from build123d import *

# Parameters (mm, degrees)
F0_R     = 25
F1_DEPTH = 1.2


with BuildPart() as f1:
    # F0 (on Top) → F1 (new body)
    with BuildSketch(Plane.XY):
        Circle(F0_R)
        Polygon((5, 15), (5, 5), (15, 5), (15, -5), (5, -5), (5, -15), (-5, -15), (-5, -5), (-15, -5), (-15, 5), (-5, 5), (-5, 15), align=None, mode=Mode.SUBTRACT)
    extrude(amount=F1_DEPTH)


solid = f1.part
For this review, take the finished solid that the model builds, in its own axes (mm). A direction names the side the tool comes from. Give positions to 0.01 mm unless a question says otherwise; leave off trailing zeros. Order: outer loops, then holes, each group sorted by start corner. A loop starts at its lowest first (then second) coordinate and runs counter-clockwise, first axis right, second up. Notation, with made-up numbers: M 61,81 L 83,81 A17 ccw 83,100 Z; hole C 80,63.25 d1. An arc over 180 degrees is marked long. Answer in a Markdown table with one row per item. Add a question column.
(1) Consider section C-C on z = 0.8. State the section outline as (x, y) points, and give its area (3 significant figures).
(2) For faces 1 (the face through (0, -15, 1)), 2 (the face through (5.2, -5.2, 0)), list the 3-axis set-ups (+Z, -Z, +X, -X, +Y, -Y) from which the entire face can be reached by the end or side of a thin tool; tool diameter is ignored.
(3) Wall thickness on probe 1 along X at (y, z) = (0.5, 1.05) (3 decimals); probe 2 along X at (y, z) = (2, 1.15); probe 3 along Y at (x, z) = (-3, 1.1): over which ranges is each line inside the solid? List them lowest first. Write a range as [from, to].
(4) Mouldability with a two-part tool opening along Y and no side actions: class faces 3 (the face through (5.2, -5.2, 1.2)), 4 (the face through (23.846, 7.509, 0.592)), 5 (the face through (-10, -5, 1)) as +Y half, -Y half, draft (parallel to the pull), parting line (faces both ways), or undercut.
(5) Consider section D-D on x = -18. State the section outline as (y, z) points, and give its area (3 significant figures).
(6) Consider section A-A on y = 0. State the section outline as (x, z) points.
(7) For pin 1 (2 mm diameter, centred on x = -4, y = 3, fed in from -Z); pin 2 (0.6 mm diameter, centred on y = -1.5, z = 1, fed in from -X); pin 3 (10 mm diameter, centred on x = 16.5, y = 16.5, fed in from -Z); pin 4 (0.6 mm diameter, centred on y = -10.5, z = 1, fed in from +X), all flat-tipped, find the tip position at first contact; note any pin that passes through.
Evaluation:
| question | item | result |
|---|---|---|
| 1 | outline | C 0,0 d50; hole M -15,-5 L -5,-5 L -5,-15 L 5,-15 L 5,-5 L 15,-5 L 15,5 L 5,5 L 5,15 L -5,15 L -5,5 L -15,5 Z |
| 1 | area | 1,460 mm^2 |
| 2 | face 1 | +Z, -Z |
| 2 | face 2 | -Z, +X, -X, +Y, -Y |
| 3 | probe 1 | x = [-24.995, -15], [15, 24.995] |
| 3 | probe 2 | x = [-24.92, -15], [15, 24.92] |
| 3 | probe 3 | y = [-24.82, -15], [15, 24.82] |
| 4 | face 3 | draft |
| 4 | face 4 | parting line |
| 4 | face 5 | undercut |
| 5 | outline | M -17.35,0 L 17.35,0 L 17.35,1.2 L -17.35,1.2 Z |
| 5 | area | 41.6 mm^2 |
| 6 | outline | M -25,0 L -15,0 L -15,1.2 L -25,1.2 Z; M 15,0 L 25,0 L 25,1.2 L 15,1.2 Z |
| 7 | pin 1 | passes through |
| 7 | pin 2 | stops at x = -24.97 |
| 7 | pin 3 | stops at z = 0 |
| 7 | pin 4 | stops at x = 22.82 |
